from build123d import *

# Parameters (mm, degrees)
SKETCH1_R           = 1.7
BOSS_EXTRUDE2_DEPTH = 4
BOSS_EXTRUDE3_DEPTH = 15


with BuildPart() as part:
    # Sketch1 → Boss-Extrude2 (new body)
    with BuildSketch(Plane(origin=(0, 0, 0), x_dir=(1, 0, 0), z_dir=(0, 1, 0))):
        with BuildLine():
            Line((-11.023477569, 2.96663632), (-11.023477569, -4.03336368))
            Line((-11.023477569, -4.03336368), (-14.338233671, -4.03336368))
            ThreePointArc((-14.338233671, -4.03336368), (-17.838233671, -0.53336368), (-14.338233671, 2.96663632))
            Line((-14.338233671, 2.96663632), (-11.023477569, 2.96663632))
        make_face()
        with Locations(Location((-13.963477569, -0.00336368, 0), (0, 0, 270))):
            Circle(SKETCH1_R, mode=Mode.SUBTRACT)
    extrude(amount=BOSS_EXTRUDE2_DEPTH)

    # Sketch2 → Boss-Extrude3 (add)
    with BuildSketch(Plane(origin=(0, 0, 0), x_dir=(1, 0, 0), z_dir=(0, 1, 0))):
        with BuildLine():
            Line((-11.023477569, 2.96663632), (-11.023477569, 4.517571778))
            Line((-11.023477569, 4.517571778), (-14.103477569, 4.517571778))
            ThreePointArc((-14.103477569, 4.517571778), (-19.899728462, -1.507895951), (-14.103477569, -7.53336368))
            Line((-14.103477569, -7.53336368), (-9.023477569, -7.53336368))
            Line((-9.023477569, -7.53336368), (-9.023477569, -4.03336368))
            Line((-9.023477569, -4.03336368), (-11.023477569, -4.03336368))
            Line((-11.023477569, -4.03336368), (-14.338233671, -4.03336368))
            ThreePointArc((-14.338233671, -4.03336368), (-17.838233671, -0.53336368), (-14.338233671, 2.96663632))
            Line((-14.338233671, 2.96663632), (-11.023477569, 2.96663632))
        make_face()
    extrude(amount=BOSS_EXTRUDE3_DEPTH)


solid = part.part
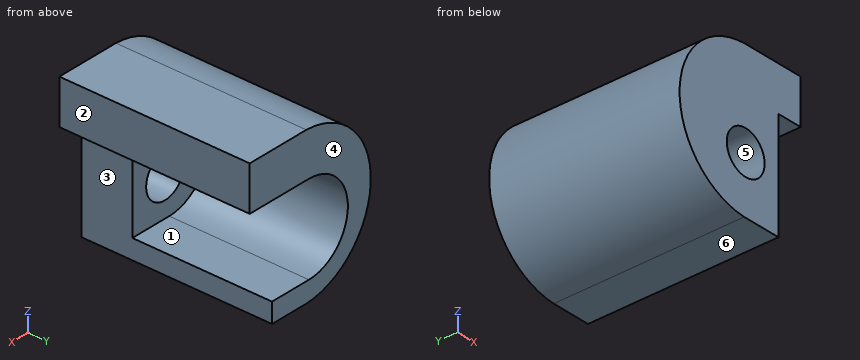
The model under review builds one solid part; all positions refer to its coordinate system, in mm. Face numbers are marked on the shaded views. A direction names the side the tool comes from. Coordinates: 2 decimals unless noted, no trailing zeros. Order: outer loops, then holes, each group sorted by start corner. A loop starts at its lowest first (then second) coordinate and runs counter-clockwise, first axis right, second up. Notation, with made-up numbers: (81, -32.75) -> (132, -32.75) arc R20 cw to (132, -23.75) -> close; hole circle Ø7 at (1.25, -40). An arc over 180 degrees is marked (long way). Answer in a Markdown table with one row per item.
(1) Insertion check: pin 1 (4 mm diameter, centred on y = 9, z = -0.5, fed in from +X); pin 2 (5.5 mm diameter, centred on x = -14, z = 0.5, fed in from +Y); pin 3 (2.5 mm diameter, centred on y = 10, z = 1.5, fed in from +X); pin 4 (3 mm diameter, centred on x = -13.96, z = 0, fed in from +Y). Each pin has a flat end and moves straight along its axis. Give the tip position at first contact, or say it passes through.
Answers:
| item | result |
|---|---|
| pin 1 | x = -16.08 |
| pin 2 | y = 4 |
| pin 3 | x = -17.05 |
| pin 4 | through |
(2) Consider section D-D (y = 2.5). Write out the cut boundary in (x, z).
Answers:
| item | result |
|---|---|
| outline | (-14.1, -4.52) -> (-11.02, -4.52) -> (-11.02, 4.03) -> (-9.02, 4.03) -> (-9.02, 7.53) -> (-14.1, 7.53) arc R6.03 ccw to start; hole circle Ø3.4 at (-13.96, 0) |
(3) The part is to be moulded in two halves that separate along Z. For the marked faces 4, 5 and 6, say which applies: +Z half, -Z half, draft (parallel to the pull), parting line (faces both ways), or undercut.
Answers:
| item | result |
|---|---|
| face 4 | draft |
| face 5 | undercut |
| face 6 | -Z half |
(4) Consider section C-C (x = -12.75). Write out the cut boundary in (y, z), plus the area to 3 significant figures.
Answers:
| item | result |
|---|---|
| outline | (0, -4.52) -> (15, -4.52) -> (15, -2.97) -> (4, -2.97) -> (4, -1.19) -> (0, -1.19) -> close; (0, 1.19) -> (4, 1.19) -> (4, 4.03) -> (15, 4.03) -> (15, 7.53) -> (0, 7.53) -> close |
| area | 94.2 mm² |
(5) Consider section A-A (z = 0.75). Write out the cut boundary in (x, y), plus the area to 3 significant figures.
Answers:
| item | result |
|---|---|
| outline | (-19.85, 0) -> (-15.49, 0) -> (-15.49, 4) -> (-17.83, 4) -> (-17.83, 15) -> (-19.85, 15) -> close; (-12.44, 0) -> (-11.02, 0) -> (-11.02, 4) -> (-12.44, 4) -> close |
| area | 45.3 mm² |
(6) Consider section B-B (y = 9). Write out the cut boundary in (x, z), plus the area to 3 significant figures.
Answers:
| item | result |
|---|---|
| outline | (-14.34, -2.97) arc R3.5 cw to (-14.34, 4.03) -> (-9.02, 4.03) -> (-9.02, 7.53) -> (-14.1, 7.53) arc R6.03 ccw to (-14.1, -4.52) -> (-11.02, -4.52) -> (-11.02, -2.97) -> close |
| area | 56.0 mm² |
(7) Wall thickness on line 1 along Z through (x, y) = (-11.75, 10.25); line 2 along Z through (x, y) = (-15.5, 9.25); line 3 along Z through (x, y) = (-10.75, 7): over which ranges is each line inside the solid? List them lowest first.
Answers:
| item | result |
|---|---|
| line 1 | -4.52 to -2.97, 4.03 to 7.53 |
| line 2 | -4.3 to -2.77, 3.83 to 7.31 |
| line 3 | 4.03 to 7.53 |
(8) Machinability: for the marked faces 1, 2 and 3, which of the approach directions +Z, -Z, +X, -X, +Y, -Y give a long, thin tool a straight path to every point of the face, cutting with its end or side? Answer none if there is none.
Answers:
| item | result |
|---|---|
| face 1 | +X, +Y |
| face 2 | +Z, -Z, +X, +Y, -Y |
| face 3 | -Z, +X, +Y, -Y |
